Input: part model. Units: mm. Frame: model coordinates. A direction names the side the tool comes from. Coordinates: 2 decimals unless noted, no trailing zeros. Write each loop counter-clockwise with the first axis right and the second up, starting at its lowest first coordinate (ties: lowest second). Pieces come first, ordered by that corner, then holes.
from build123d import *

# Parameters (mm, degrees)
SKETCH1_W           = 30
SKETCH1_H           = 12
BOSS_EXTRUDE1_DEPTH = 20
BOSS_EXTRUDE2_DEPTH = 2
SKETCH3_W           = 30
SKETCH3_H           = 12
BOSS_EXTRUDE3_DEPTH = 4
BOSS_EXTRUDE4_DEPTH = 3.5
SKETCH5_R           = 2.75
BOSS_EXTRUDE5_DEPTH = 4
FILLET1_R           = 1


with BuildPart() as part:
    # Sketch1 → Boss-Extrude1 (new body)
    with BuildSketch(Plane(origin=(0, 0, 0), x_dir=(1, 0, 0), z_dir=(0, 1, 0))):
        Rectangle(SKETCH1_W, SKETCH1_H)
    extrude(amount=BOSS_EXTRUDE1_DEPTH)

    # Sketch2 → Boss-Extrude2 (add)
    with BuildSketch(Plane(origin=(0, 20, 0), x_dir=(1, 0, 0), z_dir=(0, 1, 0))):
        with BuildLine():
            Line((-20.25, 6), (20.25, 6))
            Line((20.25, 6), (20.25, 1.414213562))
            ThreePointArc((20.25, 1.414213562), (16.25, 0), (20.25, -1.414213562))
            Line((20.25, -1.414213562), (20.25, -6))
            Line((20.25, -6), (-20.25, -6))
            Line((-20.25, -6), (-20.25, -1.414213562))
            ThreePointArc((-20.25, -1.414213562), (-16.25, 0), (-20.25, 1.414213562))
            Line((-20.25, 1.414213562), (-20.25, 6))
        make_face()
    extrude(amount=BOSS_EXTRUDE2_DEPTH)

    # Sketch3 → Boss-Extrude3 (add)
    with BuildSketch(Plane(origin=(0, 22, 0), x_dir=(1, 0, 0), z_dir=(0, 1, 0))):
        Rectangle(SKETCH3_W, SKETCH3_H)
    extrude(amount=BOSS_EXTRUDE3_DEPTH)

    # Sketch4 → Boss-Extrude4 (add)
    with BuildSketch(Plane(origin=(0, 26, 0), x_dir=(1, 0, 0), z_dir=(0, 1, 0))):
        with BuildLine():
            Line((-8.605551275, 6), (-1.394448725, 6))
            ThreePointArc((-1.394448725, 6), (-0.546683534, 5.400738139), (0.203125, 4.682679813))
            ThreePointArc((0.203125, 4.682679813), (5.75, 0), (0.203125, -4.682679813))
            ThreePointArc((0.203125, -4.682679813), (-0.546683534, -5.400738139), (-1.394448725, -6))
            Line((-1.394448725, -6), (-8.605551275, -6))
            ThreePointArc((-8.605551275, -6), (-12, 0), (-8.605551275, 6))
        make_face()
    extrude(amount=BOSS_EXTRUDE4_DEPTH)

    # Sketch5 → Boss-Extrude5 (add)
    with BuildSketch(Plane(origin=(0, 29.5, 0), x_dir=(1, 0, 0), z_dir=(0, 1, 0))):
        with Locations(Location((-5, 0, 0), (0, 0, 270))):
            Circle(SKETCH5_R)
    extrude(amount=BOSS_EXTRUDE5_DEPTH)

    # Fillet1
    fillet1_edges = [part.edges().sort_by_distance(p)[0] for p in [
        (20.25, 21, 6),
        (20.25, 21, -6),
        (-20.25, 21, -6),
        (-20.25, 21, 6),
        (15, 24, 6),
        (15, 24, -6),
        (-15, 24, -6),
        (-15, 24, 6),
        (0, 0, 6),
        (-15, 0, 0),
        (0, 0, -6),
        (15, 0, 0),
        (15, 10, 6),
        (-15, 10, 6),
        (-15, 10, -6),
        (15, 10, -6),
    ]]
    fillet(fillet1_edges, radius=FILLET1_R)


solid = part.part
Item 1: Pin query (flat end, axial travel): pin 1 Ø1.2 at (y, z) = (24.5, -1) entering from +X; pin 2 Ø1.9 at (x, z) = (17, -1.5) entering from -Y; pin 3 Ø5 at (y, z) = (14.5, -2.5) entering from -X. Return the tip coordinate at first contact, or that it passes through.
Item 2: Section query C-C, the plane x = -5. Return loops of the section in (y, z).
Item 3: Section query D-D, the plane y = 14. Return loops of the section in (x, z).
Item 4: Section query A-A, the plane x = -18.5. Return loops of the section in (y, z).
Item 5: Access query for faces 1 (the face through (14.699, 24.028, -5.715)), 2 (the face through (14.715, 24.028, 5.699)), 3 (the face through (15, 10, 0)). Directions: +Z, -Z, +X, -X, +Y, -Y. A direction counts if a zero-diameter tool reaches every point of the face in a straight line with its end or side. Return the directions, or none.
Item 6: Section query B-B, the plane z = 0. Return loops of the section in (x, y), then the cut area to 3 significant figures.
Item 7: Material intervals for line 1 (Z direction, x = 18.5, y = 20.65); line 2 (Y direction, x = 9.5, z = -4); line 3 (Y direction, x = -8.5, z = -3.25), sorted ascending.
The answers:
1. pin 1: stops at x = 15
1. pin 2: stops at y = 20
1. pin 3: stops at x = -15
2. outline: (0, -5) arc R1 ccw to (1, -6) - (29.5, -6) - (29.5, -2.75) - (33.5, -2.75) - (33.5, 2.75) - (29.5, 2.75) - (29.5, 6) - (1, 6) arc R1 ccw to (0, 5) - close
3. outline: (-15, -5) arc R1 ccw to (-14, -6) - (14, -6) arc R1 ccw to (15, -5) - (15, 5) arc R1 ccw to (14, 6) - (-14, 6) arc R1 ccw to (-15, 5) - close
4. outline: (20, -6) - (22, -6) - (22, -2.25) - (20, -2.25) - close; (20, 2.25) - (22, 2.25) - (22, 6) - (20, 6) - close
5. face 1: -Z, +X, +Y
5. face 2: +Z, +X, +Y
5. face 3: +Z, -Z, +X, -Y
6. outline: (-16.25, 20) - (-15, 20) - (-15, 1) arc R1 ccw to (-14, 0) - (14, 0) arc R1 ccw to (15, 1) - (15, 20) - (16.25, 20) - (16.25, 22) - (15, 22) - (15, 26) - (5.75, 26) - (5.75, 29.5) - (-2.25, 29.5) - (-2.25, 33.5) - (-7.75, 33.5) - (-7.75, 29.5) - (-12, 29.5) - (-12, 26) - (-15, 26) - (-15, 22) - (-16.25, 22) - close
6. area: 869 mm2
7. line 1: z = -6 to -2.25, 2.25 to 6
7. line 2: y = 0 to 26
7. line 3: y = 0 to 29.5
